from build123d import *

# Parameters (mm, degrees)
SKETCH1_R           = 13
SKETCH1_R_2         = 11.5
BOSS_EXTRUDE5_DEPTH = 45
BOSS_EXTRUDE7_DEPTH = 3


with BuildPart() as part:
    # Sketch1 → Boss-Extrude5 (new body)
    with BuildSketch(Plane(origin=(0, 0, 0), x_dir=(0, 0, -1), z_dir=(1, 0, 0))):
        Circle(SKETCH1_R)
        Circle(SKETCH1_R_2, mode=Mode.SUBTRACT)
    extrude(amount=BOSS_EXTRUDE5_DEPTH)

    # Sketch5 → Boss-Extrude7 (add)
    with BuildSketch(Plane.ZY):
        with BuildLine():
            Line((-10, 15), (10, 15))
            ThreePointArc((10, 15), (13.535533906, 13.535533906), (15, 10))
            Line((15, 10), (15, -10))
            ThreePointArc((15, -10), (13.535533906, -13.535533906), (10, -15))
            Line((10, -15), (-10, -15))
            ThreePointArc((-10, -15), (-13.535533906, -13.535533906), (-15, -10))
            Line((-15, -10), (-15, 10))
            ThreePointArc((-15, 10), (-13.535533906, 13.535533906), (-10, 15))
        make_face()
    extrude(amount=BOSS_EXTRUDE7_DEPTH)


solid = part.part
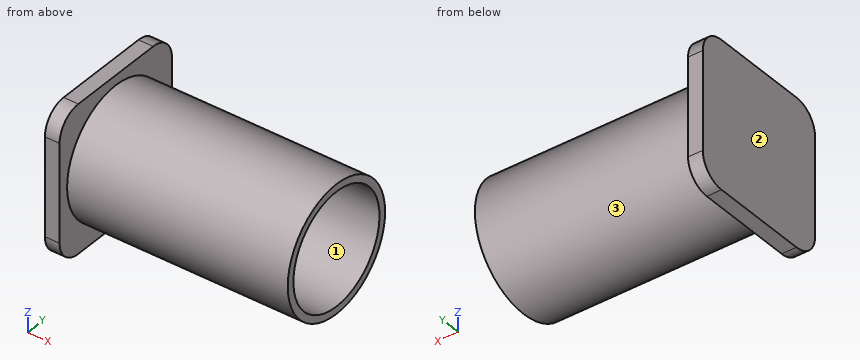
Could you check a few things on this model? Use its own coordinates, in mm. Face numbers are marked on the shaded views. Give positions to 0.01 mm unless a question says otherwise; leave off trailing zeros. Order: outer loops, then holes, each group sorted by start corner. A loop starts at its lowest first (then second) coordinate and runs counter-clockwise, first axis right, second up.
1. Suppose I cut it at C-C (x = 12). List the corners of the cut face in (y, z) for me, plus the area to 3 significant figures.
2. We'd pull the mould along Z, two halves only. Please class the marked faces 1, 2 and 3: pulls with the +Z half, pulls with the -Z half, needs draft (parallel to the pull), parting line crosses it, or undercut.
3. Suppose I cut it at A-A (y = 7). List the corners of the cut face in (x, z) for me, plus the area to 3 significant figures.
4. Will these pins go through, and if not, where does the flat tip stop? P1, Ø5, axis at x = 23.5, y = 12, coming from the +Z side; P2, Ø3, axis at x = 9.5, z = -6.5, coming from the +Y side; P3, Ø1, axis at x = 27, z = -4, coming from the -Y side.
5. I need wall thicknesses on L1, parallel to Y at x = 11, z = 0; L2, parallel to X at y = 8.75, z = 10.25; L3, parallel to Z at x = 29.5, y = -7.5. Which ranges of each line are inside material? Lowest first, please.
6. Suppose I cut it at B-B (z = 0). List the corners of the cut face in (x, y) for me, plus the area to 3 significant figures.
Solved:
1. outline: circle Ø26 at (0, 0); hole circle Ø23 at (0, 0)
1. area: 115 mm2
2. face 1: undercut
2. face 2: needs draft
2. face 3: parting line crosses it
3. outline: (-3, -15) - (0, -15) - (0, -10.95) - (45, -10.95) - (45, -9.12) - (0, -9.12) - (0, 9.12) - (45, 9.12) - (45, 10.95) - (0, 10.95) - (0, 15) - (-3, 15) - close
3. area: 255 mm2
4. P1: stops at z = 8.87
4. P2: stops at y = 12
4. P3: stops at y = -12.52
5. L1: y = -13 to -11.5, 11.5 to 13
5. L2: x = -3 to 0
5. L3: z = -10.62 to -8.72, 8.72 to 10.62
6. outline: (-3, -15) - (0, -15) - (0, -13) - (45, -13) - (45, -11.5) - (0, -11.5) - (0, 11.5) - (45, 11.5) - (45, 13) - (0, 13) - (0, 15) - (-3, 15) - close
6. area: 225 mm2
